Can you work these out from the drawing? Everything is in mm from the part's minimum corner. Round coordinates to 2 decimals unless told otherwise and drop trailing zeros. Loops run counter-clockwise (first coordinate to the right, second up) from the corner with the lowest first, then second, coordinate; pieces in that order, holes last. Notation, with made-up numbers: (68.5, 61.25) - (98.5, 61.25) arc R17 cw to (98.5, 89.25) - close; hole circle Ø2 at (40, 27.25). An arc over 180 degrees is marked (long way). Put each result on its own line as item: value. Start each with the question number.
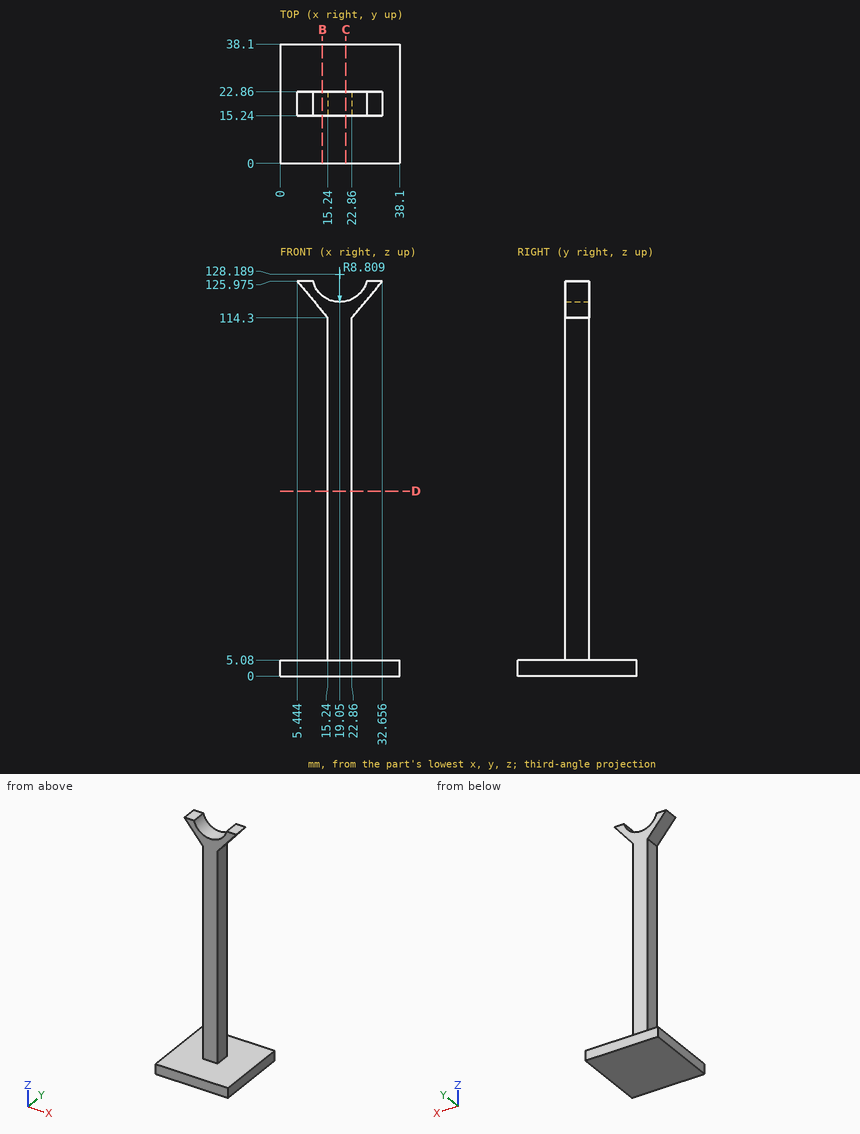
Item 1: Suppose I cut it at B-B, the plane x = 13.5. List the corners of the cut face in (y, z) for me.
Item 2: Suppose I cut it at C-C, the plane x = 21. List the corners of the cut face in (y, z) for me, then the cut area to 3 significant figures.
Item 3: Will these pins go through, and if not, where does the flat tip stop? P1, Ø12, axis at y = 19.5, z = 41.5, coming from the +X side; P2, Ø11.5, axis at x = 16, y = 26, coming from the +Z side (1 decimal); P3, Ø6, axis at x = 19, z = 105, coming from the +Y side.
Item 4: Suppose I cut it at D-D, the plane z = 59. List the corners of the cut face in (x, y) for me.
Item 5: I need wall thicknesses on line 1 (Z direction, x = 15.5, y = 10); line 2 (Y direction, x = 20.5, z = 20.5). Which ranges of each line are inside material? Lowest first, please. Write a range as from..to.
Numbers:
1. outline: (0, 0) - (38.1, 0) - (38.1, 5.08) - (0, 5.08) - close; (15.24, 116.37) - (22.86, 116.37) - (22.86, 121.35) - (15.24, 121.35) - close
2. outline: (0, 0) - (38.1, 0) - (38.1, 5.08) - (22.86, 5.08) - (22.86, 119.6) - (15.24, 119.6) - (15.24, 5.08) - (0, 5.08) - close
2. area: 1,070 mm^2
3. P1: x = 22.86
3. P2: z = 124.2
3. P3: y = 22.86
4. outline: (15.24, 15.24) - (22.86, 15.24) - (22.86, 22.86) - (15.24, 22.86) - close
5. line 1: 0..5.08
5. line 2: 15.24..22.86
